Autodesk Inventor part; units mm, degrees
ref_plane "Arbeitsebene1" through (-9, -9, -7.8) normal (0, 0, -1) x (0, 1, 0)
ref_plane "YZ Plane" through (0, 0, 0) normal (1, 0, 0) x (0, 1, 0)
ref_plane "XZ Plane" through (0, 0, 0) normal (0, 1, 0) x (-1, 0, 0)
sketch "Skizze1" plane through (0, 0, 0) normal (0, 0, 1) x (1, 0, 0)
  arc A0 (-9, -8) -> (-8, -9) centre (-8, -8) ccw
  line L0 (8, -9) -> (-8, -9)
  arc A1 (8, -9) -> (9, -8) centre (8, -8) ccw
  line L1 (9, 8) -> (9, -8)
  arc A2 (9, 8) -> (8, 9) centre (8, 8) ccw
  line L2 (-8, 9) -> (8, 9)
  arc A3 (-8, 9) -> (-9, 8) centre (-8, 8) ccw
  line L3 (-9, -8) -> (-9, 8)
  circle A4 centre (0, 0) radius 5.8
  arc A5 (-8, 9.1) -> (-9.1, 8) centre (-8, 8) ccw
  line L4 (-8, 9.1) -> (8, 9.1)
  arc A6 (9.1, 8) -> (8, 9.1) centre (8, 8) ccw
  line L5 (9.1, 8) -> (9.1, -8)
  arc A7 (8, -9.1) -> (9.1, -8) centre (8, -8) ccw
  line L6 (8, -9.1) -> (-8, -9.1)
  arc A8 (-9.1, -8) -> (-8, -9.1) centre (-8, -8) ccw
  line L7 (-9.1, -8) -> (-9.1, 8)
  line L8 (14, 14) -> (-14, 14)
  line L9 (-14, 14) -> (-14, -14)
  line L10 (-14, -14) -> (14, -14)
  line L11 (14, -14) -> (14, 14)
  line L12 (14, 14) -> (-14, -14) construction
  line L13 (-14, 14) -> (14, -14) construction
  point P0 (0, 0)
  dimension "d0" = 0.1
  dimension "d1" = 28
  dimension "d2" = 28
ref_plane "Arbeitsebene1" through (-9, -9, -7.8) normal (0, 0, -1) x (0, 1, 0)
extrude "Extrusion1" add sketch "Skizze1" against normal up to surface (7.8 mm away) contours L11 L10 L9 L8
sketch "Skizze2" plane through (0, 0, 0) normal (0, 0, 1) x (1, 0, 0)
  line L0 (-14, 14) -> (-14, -14)
  line L1 (-14, -14) -> (14, -14)
  line L2 (14, -14) -> (14, 14)
  line L3 (14, 14) -> (-14, 14)
  line L4 (9.1, 8) -> (9.1, -8)
  arc A0 (8, -9.1) -> (9.1, -8) centre (8, -8) ccw
  line L5 (8, -9.1) -> (-8, -9.1)
  arc A1 (-9.1, -8) -> (-8, -9.1) centre (-8, -8) ccw
  line L6 (-9.1, -8) -> (-9.1, 8)
  arc A2 (-8, 9.1) -> (-9.1, 8) centre (-8, 8) ccw
  line L7 (-8, 9.1) -> (8, 9.1)
  arc A3 (9.1, 8) -> (8, 9.1) centre (8, 8) ccw
  line L8 (-7.6, 7.6) -> (-7.6, -7.6)
  line L9 (-7.6, -7.6) -> (7.6, -7.6)
  line L10 (7.6, -7.6) -> (7.6, 7.6)
  line L11 (7.6, 7.6) -> (-7.6, 7.6)
  point P0 (0, 0)
  dimension "d5" = 1.5
extrude "Extrusion2" add sketch "Skizze2" along normal blind 0.5 contours L3 L2 L1 L0 | L4 A0 L5 A1 L6 A2 L7 A3 | L11 L10 L9 L8
sketch "Skizze3" plane through (0, 0, 0.5) normal (0, 0, 1) x (1, 0, 0)
  line L0 (-14, -14) -> (14, -14)
  line L1 (14, -14) -> (14, 14)
  line L2 (14, 14) -> (-14, 14)
  line L3 (-14, 14) -> (-14, -14)
  circle A0 centre (0, 3.1887) radius 4
  dimension "d8" = 8
extrude "Extrusion3" add sketch "Skizze3" along normal blind 3
sketch "Skizze4" plane through (0, 0, 3.5) normal (0, 0, 1) x (1, 0, 0)
  line L0 (14, -14) -> (14, 14)
  line L1 (14, 14) -> (-14, 14)
  line L2 (-14, 14) -> (-14, -14)
  line L3 (-14, -14) -> (14, -14)
  circle A0 centre (0, 3.1887) radius 4
  line L4 (5, -10.8) -> (-5, -10.8)
  line L5 (-14, 14) -> (-14, -14)
  line L6 (14, -14) -> (-14, -14)
  line L7 (-14, -14) -> (-14, -9.3)
  line L8 (-14, -9.3) -> (14, -9.3)
  line L9 (14, -9.3) -> (14, -14)
  line L10 (-14, 14) -> (-12.5, 14)
  line L11 (-12.5, 14) -> (-12.5, -9.3)
  line L12 (-12.5, -9.3) -> (-14, -9.3)
  line L13 (-14, -9.3) -> (-14, 14)
  line L14 (14, -14) -> (14, 14)
  line L15 (14, 14) -> (12.5, 14)
  line L16 (12.5, 14) -> (12.5, -9.3)
  line L17 (12.5, -9.3) -> (14, -9.3)
  line L18 (14, -9.3) -> (14, 14)
  point P0 (0, 0)
  point P1 (14, -9.3)
  point P2 (12.5, 14)
  dimension "d11" = 1.5
  dimension "d22" = 1.5
  dimension "d23" = 1.5
extrude "Extrusion4" cut sketch "Skizze4" against normal through all contours L3 L2 L8 L0 | L8 L16 L1 L0 | L2 L1 L11 L8
sketch "Skizze5" plane through (0, 0, 3.5) normal (0, 0, 1) x (1, 0, 0)
  circle A0 centre (-9, 11.7) radius 2
  circle A1 centre (-9, -3.3) radius 2.5019
  line L0 (-9, -3.3) -> (9, -3.3)
  line L1 (9, -3.3) -> (9, 6.7)
  line L2 (9, 6.7) -> (-9, 6.7)
  line L3 (-9, 6.7) -> (-9, -3.3)
  dimension "d25" = 18
hole "Bohrung1" at (9, -3.3, 3.5) at (9, 6.7, 3.5) at (-9, -3.3, 3.5) at (-9, 11.7, 3.5) direction (0, 0, -1) diameter 3 depth 0.0001 tip angle 140
sketch "Skizze6" plane through (0, 0, 3.5) normal (0, 0, 1) x (1, 0, 0)
  circle A0 centre (-9, 11.7) radius 1.5
  circle A1 centre (-9, 11.7) radius 2.5
  point P0 (0, 0)
  dimension "d26" = 5
extrude "Extrusion5" cut sketch "Skizze6" against normal blind 4 contours A0 | A1
properties part number "10_SOOCT_VCM_Mount_v0"
Geometry: final body of the model. Coordinates: model frame, mm. A direction names the side the tool comes from. Coordinates: 2 decimals unless noted, no trailing zeros. Order: outer loops, then holes, each group sorted by start corner. A loop starts at its lowest first (then second) coordinate and runs counter-clockwise, first axis right, second up. Notation, with made-up numbers: M 51.5,-16.75 L 60.5,-16.75 A17 ccw 60.5,6.25 Z; hole C 36.25,44 d6. An arc over 180 degrees is marked long. Answer in a Markdown table with one row per item. Add a question column.
Q1. Section query B-B on y = 11.7. Return the cut outline in (x, z).
Q2. Reachability of faces 1 (the flat face through (12.5, 3, -2)), 2 (the cylindrical face through (3.815, 1.987, 1.979)), 3 (the flat face through (0, 9.1, -4)) from +Z, -Z, +X, -X, +Y, -Y: full face, straight path, thin tool, end or side. Return the list, or none.
Q3. Line query: L1, parallel to Y at x = 2.25, z = -5.5; L2, parallel to X at y = 11.7, z = 0.7; L3, parallel to X at y = 6.5, z = -2.5. Output: solid intervals per line, ascending.
Q4. Mould query, pull axis Y, two halves, no side actions, for faces 4 (the flat face through (0, 10, -7.8)), 5 (the flat face through (9.1, 0, -4)). Classes: released by +Y, released by -Y, zero draft, split by the parting line, or undercut.
Q5. Contact query for flat-ended pins moving along their axis: P1, Ø1.4, axis at x = -8.5, y = 10.5, coming from the +Z side; P2, Ø9, axis at x = 0, y = 3.19, coming from the -Z side; P3, Ø2.5, axis at x = -1.5, y = 4.5, coming from the +Z side. Output: stop coordinate, or through.
Q6. Section query C-C on x = 0. Return the cut outline in (y, z), and give its area (3 significant figures).
Q7. Section query D-D on y = 0.25. Return the cut outline in (x, z).
Q8. Section query A-A on z = -4. Return the cut outline in (x, y).
Completed:
| question | item | result |
|---|---|---|
| 1 | outline | M -12.5,-7.8 L 12.5,-7.8 L 12.5,3.5 L -6.5,3.5 L -6.5,-0.5 L -11.5,-0.5 L -11.5,3.5 L -12.5,3.5 Z |
| 2 | face 1 | +Z, -Z, +X, +Y, -Y |
| 2 | face 2 | +Z |
| 2 | face 3 | -Z |
| 3 | L1 | y = -9.3 to -9.1, 9.1 to 14 |
| 3 | L2 | x = -12.5 to -11.5, -6.5 to 12.5 |
| 3 | L3 | x = -12.5 to -9.1, 9.1 to 12.5 |
| 4 | face 4 | zero draft |
| 4 | face 5 | undercut |
| 5 | P1 | stops at z = -0.5 |
| 5 | P2 | stops at z = 0 |
| 5 | P3 | stops at z = 0.5 |
| 6 | outline | M -9.3,-7.8 L -9.1,-7.8 L -9.1,0 L 9.1,0 L 9.1,-7.8 L 14,-7.8 L 14,3.5 L 7.19,3.5 L 7.19,0.5 L -0.81,0.5 L -0.81,3.5 L -9.3,3.5 Z |
| 6 | area | 97.3 mm2 |
| 7 | outline | M -12.5,-7.8 L -9.1,-7.8 L -9.1,0 L 9.1,0 L 9.1,-7.8 L 12.5,-7.8 L 12.5,3.5 L 2.71,3.5 L 2.71,0.5 L -2.71,0.5 L -2.71,3.5 L -12.5,3.5 Z |
| 8 | outline | M -12.5,-9.3 L 12.5,-9.3 L 12.5,14 L -12.5,14 Z; hole M -9.1,-8 A1.1 ccw -8,-9.1 L 8,-9.1 A1.1 ccw 9.1,-8 L 9.1,8 A1.1 ccw 8,9.1 L -8,9.1 A1.1 ccw -9.1,8 Z |
